Could you check a few things on this model? Use its own coordinates, in mm. A direction names the side the tool comes from. Give positions to 0.01 mm unless a question says otherwise; leave off trailing zeros. Write each loop counter-clockwise with the first axis right and the second up, starting at its lowest first coordinate (ties: lowest second). Pieces come first, ordered by that corner, then holes. Notation, with made-up numbers: M 21,32 L 59,32 A6 ccw 59,42 Z; hole C -27.75,30.25 d5. An arc over 180 degrees is marked long. One line per item, written item: value.
```python
from build123d import *

# Parameters (mm, degrees)
SKETCH1_R               = 75
BOSS_EXTRUDE1_DEPTH     = 10
SKETCH2_R               = 45
SKETCH2_R_2             = 40
BOSS_EXTRUDE2_DEPTH     = 50
SKETCH5_W               = 75
SKETCH5_H               = 75
BOSS_EXTRUDE3_DEPTH     = 50
CUT_EXTRUDE2_DEPTH      = 103
CUT_EXTRUDE3_DEPTH      = 103
CUT_EXTRUDE3_DEPTH_BACK = 103
SKETCH9_W               = 20
SKETCH9_H               = 50
CUT_EXTRUDE4_DEPTH      = 103
CUT_EXTRUDE4_DEPTH_BACK = 103
SKETCH10_R              = 5
CUT_EXTRUDE5_DEPTH      = 103
SKETCH11_R              = 5
SKETCH13_W              = 1000
SKETCH13_H              = 1000
BOSS_EXTRUDE4_DEPTH     = 4


with BuildPart() as part:
    # Sketch1 → Boss-Extrude1 (new body)
    with BuildSketch(Plane(origin=(0, 0, 0), x_dir=(1, 0, 0), z_dir=(0, 1, 0))):
        Circle(SKETCH1_R)
    extrude(amount=BOSS_EXTRUDE1_DEPTH)

    # Sketch2 → Boss-Extrude2 (add)
    with BuildSketch(Plane.XZ):
        Circle(SKETCH2_R)
        Circle(SKETCH2_R_2, mode=Mode.SUBTRACT)
    extrude(amount=BOSS_EXTRUDE2_DEPTH)

    # Sketch5 → Boss-Extrude3 (add)
    with BuildSketch(Plane(origin=(0, 10, 0), x_dir=(1, 0, 0), z_dir=(0, 1, 0))):
        Rectangle(SKETCH5_W, SKETCH5_H)
    extrude(amount=BOSS_EXTRUDE3_DEPTH)

    # Sketch6 → Cut-Extrude2 (cut)
    with BuildSketch(Plane.XY.offset(37.5)):
        Polygon((20, 60), (37.5, 10), (43.069722315, 10), (43.069722315, 63.034625831), (-42.678571429, 63.034625831), (-42.678571429, 10), (-37.5, 10), (-20, 60), align=None)
        Polygon((-12.90518995, 50), (-26.90518995, 10), (26.90518995, 10), (12.90518995, 50), align=None)
    extrude(amount=-CUT_EXTRUDE2_DEPTH, mode=Mode.SUBTRACT)

    # Sketch7 → Cut-Extrude3 (cut, two sides)
    with BuildSketch(Plane(origin=(0, 0, 0), x_dir=(0, 0, -1), z_dir=(1, 0, 0))) as cut_extrude3_sk:
        Polygon((20, 60), (-20, 60), (-37.5, 10), (-47.69302584, 10), (-47.69302584, 63.764621125), (47.449694076, 63.764621125), (47.449694076, 10), (37.5, 10), align=None)
    extrude(amount=CUT_EXTRUDE3_DEPTH, mode=Mode.SUBTRACT)
    extrude(cut_extrude3_sk.sketch, amount=-CUT_EXTRUDE3_DEPTH_BACK, mode=Mode.SUBTRACT)

    # Sketch9 → Cut-Extrude4 (cut, two sides)
    with BuildSketch(Plane(origin=(0, 0, 0), x_dir=(0, 0, -1), z_dir=(1, 0, 0))) as cut_extrude4_sk:
        with Locations((0, 35)):
            Rectangle(SKETCH9_W, SKETCH9_H)
    extrude(amount=CUT_EXTRUDE4_DEPTH, mode=Mode.SUBTRACT)
    extrude(cut_extrude4_sk.sketch, amount=-CUT_EXTRUDE4_DEPTH_BACK, mode=Mode.SUBTRACT)

    # Sketch10 → Cut-Extrude5 (cut)
    with BuildSketch(Plane(origin=(0, 10, 0), x_dir=(1, 0, 0), z_dir=(0, 1, 0))):
        Circle(SKETCH10_R)
    extrude(amount=-CUT_EXTRUDE5_DEPTH, mode=Mode.SUBTRACT)

    # Sweep1: sweep along a curve in space
    with BuildLine() as sweep1_path:
        Line((-60, 10, 0), (-60, 210, 0))
    # Sketch11 → Sweep1 (sweep)
    with BuildSketch(Plane(origin=(0, 10, 0), x_dir=(1, 0, 0), z_dir=(0, 1, 0))):
        with Locations((-60, 0)):
            Circle(SKETCH11_R)
        with Locations((30, 51.961524227)):
            Circle(SKETCH11_R)
        with Locations((30, -51.961524227)):
            Circle(SKETCH11_R)
    sweep(path=sweep1_path.line)

    # Sketch13 → Boss-Extrude4 (add)
    with BuildSketch(Plane(origin=(0, 210, 0), x_dir=(1, 0, 0), z_dir=(0, 1, 0))):
        Rectangle(SKETCH13_W, SKETCH13_H)
    extrude(amount=BOSS_EXTRUDE4_DEPTH)

    # Sketch17 → Revolve2 (revolve)
    with BuildSketch(Plane(origin=(0, 0, 0), x_dir=(0, 0, -1), z_dir=(1, 0, 0))):
        Polygon((10, 55), (10, 70), (5, 70), (3.237517532, 60.004465223), (-3.237517532, 60.004465223), (-5, 70), (-10, 70), (-10, 55), align=None)
    revolve(axis=Axis((0, 55, -10), (0, 0, 1)))


solid = part.part
```
1) If we section it at C-C, the plane x = -228.5: Write out the boundary of the cut face in (y, z).
Outcome:
outline: M 210,-500 L 214,-500 L 214,500 L 210,500 Z
2) Please list where these lines run through material, in increasing order: L1, parallel to X at y = 5, z = 0; L2, parallel to Z at x = 0, y = -11.5. Write a range as from..to.
Outcome:
L1: x = -75..-5, 5..75
L2: z = -45..-40, 40..45
3) I'm going to push flat-ended pins straight in: pin 1 (19 mm diameter, centred on x = 26.5, y = 32.5, fed in from +Z); pin 2 (11.5 mm diameter, centred on x = 0, z = 0, fed in from -Y); pin 3 (10 mm diameter, centred on y = 70.5, z = -60, fed in from +X). Where does each tip first touch, or does it pass through?
Outcome:
pin 1: stops at z = 56.96
pin 2: stops at y = 0
pin 3: stops at x = 33.97
4) If we section it at B-B, the plane z = 257: Write out the boundary of the cut face in (x, y).
Outcome:
outline: M -500,210 L 500,210 L 500,214 L -500,214 Z
5) We'd pull the mould along Y, two halves only. Please class faces 4 (the face through (8, 0, -1)), 5 (the face through (-8.67, -24.65, -39.05)), 6 (the face through (-19.8, 30.3, -20.5)): pulls with the +Y half, pulls with the -Y half, needs draft (parallel to the pull), parting line crosses it, or undercut.
Outcome:
face 4: pulls with the -Y half
face 5: needs draft
face 6: undercut
6) If we section it at D-D, the plane y = 177.5: Write out the boundary of the cut face in (x, z).
Outcome:
outline: C -60,0 d10; C 30,-51.96 d10; C 30,51.96 d10
7) On a 3-axis mill with a long thin cutter (end or side, diameter ignored), from which of +Z, -Z, +X, -X, +Y, -Y can I reach the whole of each face in a straight line? I mean faces 1 (the face through (-0.66, 40.015, -7.465)), 2 (the face through (16.49, 42.29, -26.2)), 3 (the face through (25, 35, 10)). Say none if no direction works.
Outcome:
face 1: none
face 2: +X, -X
face 3: +X
8) If we section it at A-A, the plane y = 22: Write out the boundary of the cut face in (x, z), then the cut area to 3 significant figures.
Outcome:
outline: C -60,0 d10; M -33.3,-33.3 L -22.71,-33.3 L -22.71,-10 L -33.3,-10 Z; M -33.3,10 L -22.71,10 L -22.71,33.3 L -33.3,33.3 Z; M 22.71,-33.3 L 33.3,-33.3 L 33.3,-10 L 22.71,-10 Z; M 22.71,10 L 33.3,10 L 33.3,33.3 L 22.71,33.3 Z; C 30,-51.96 d10; C 30,51.96 d10
area: 1,220 mm^2
